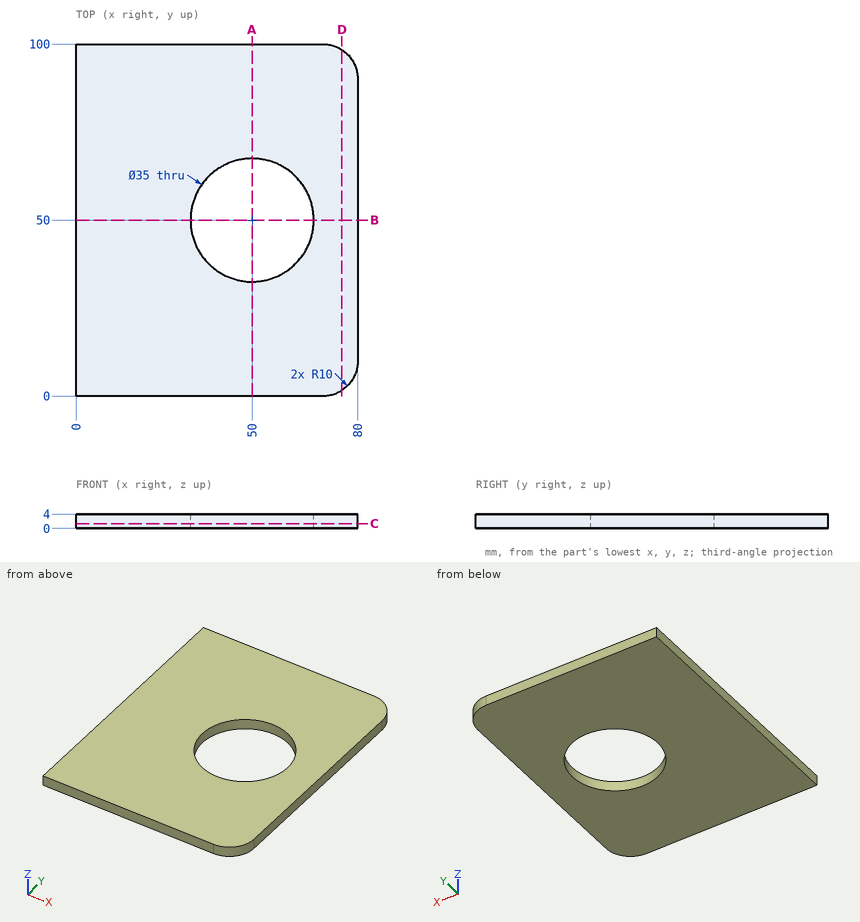
Could you check a few things on this drawing? It's one solid part, dimensions in mm from its lowest x, y, z. Round coordinates to 2 decimals unless told otherwise and drop trailing zeros. Order: outer loops, then holes, each group sorted by start corner. A loop starts at its lowest first (then second) coordinate and runs counter-clockwise, first axis right, second up. Notation, with made-up numbers: M 55,3 L 102,3 A25 ccw 102,15 Z; hole C 25,23.25 d7. An arc over 180 degrees is marked long. One line per item, written item: value.
(1) Imagine slicing it at D-D (x = 75.5). Write out the boundary of the cut face in (y, z).
Ans:
outline: M 1.65,0 L 98.35,0 L 98.35,4 L 1.65,4 Z
(2) Imagine slicing it at C-C (z = 1.3). Write out the boundary of the cut face in (x, y).
Ans:
outline: M 0,0 L 70,0 A10 ccw 80,10 L 80,90 A10 ccw 70,100 L 0,100 Z; hole C 50,50 d35
(3) I need wall thicknesses on line 1 along Y through (x, z) = (50, 2.5); line 2 along X through (y, z) = (55, 2.7); line 3 along Y through (x, z) = (39, 0.25). Which ranges of each line are inside material? Lowest first, please. Write a range as from..to.
Ans:
line 1: y = 0..32.5, 67.5..100
line 2: x = 0..33.23, 66.77..80
line 3: y = 0..36.39, 63.61..100
(4) Imagine slicing it at B-B (y = 50). Write out the boundary of the cut face in (x, z).
Ans:
outline: M 0,0 L 32.5,0 L 32.5,4 L 0,4 Z; M 67.5,0 L 80,0 L 80,4 L 67.5,4 Z
(5) Imagine slicing it at A-A (x = 50). Write out the boundary of the cut face in (y, z).
Ans:
outline: M 0,0 L 32.5,0 L 32.5,4 L 0,4 Z; M 67.5,0 L 100,0 L 100,4 L 67.5,4 Z
